```python
from build123d import *

# Parameters (mm, degrees)
F1_DEPTH = 65


# Not quite as in the source:
# - a feature names something its author has since deleted; it is built from what else it names


with BuildPart() as f1:
    # F0 (on Front) → F1 (new body)
    with BuildSketch(Plane.XZ):
        Polygon((0, 10), (0, 0), (20, 0), (20, 65), (0, 65), (0, 55), align=None)
        with BuildLine():
            ThreePointArc((13.25, 10), (10, 6.75), (6.75, 10))
            ThreePointArc((6.75, 10), (10, 13.25), (13.25, 10))
        make_face(mode=Mode.SUBTRACT)
        with BuildLine():
            ThreePointArc((13.25, 55), (10, 51.75), (6.75, 55))
            ThreePointArc((6.75, 55), (10, 58.25), (13.25, 55))
        make_face(mode=Mode.SUBTRACT)
    extrude(amount=F1_DEPTH)


solid = f1.part
```
CAD build for the part. Positions are in the model's coordinates, mm. Give positions to 0.01 mm unless a question says otherwise; leave off trailing zeros. Write each loop counter-clockwise with the first axis right and the second up, starting at its lowest first coordinate (ties: lowest second). Pieces come first, ordered by that corner, then holes. Notation, with made-up numbers: M -38.5,72 L -29.5,72 A32 ccw -29.5,108 Z; hole C 47.25,50 d5. An arc over 180 degrees is marked long. Return JSON: item names as keys, results as strings. Group by question number.
(1) Band-saw the part on B-B (y = -9). Give the cut face in (x, z), and give its area (3 significant figures).
(2) Drill centre lines: L1, parallel to Z at x = 10, y = -23.5; L2, parallel to Z at x = 12.25, y = -61.5; L3, parallel to X at y = -6, z = 13. Where is each one in solid material? Low to high. Write a range as [from, to].
(3) Mould opens along X. For faces 1 (the face through (0, -32, 33)), 2 (the face through (12.395, -32.045, 12.197)), 3 (the face through (10, -65, 33)) say: pulls with the +X half, pulls with the -X half, needs draft (parallel to the pull), parting line crosses it, or undercut.
(4) Band-saw the part on D-D (z = 57). Give the cut face in (x, y).
(5) Band-saw the part on C-C (x = 10). Give the cut face in (y, z).
(6) Band-saw the part on A-A (z = 10). Give the cut face in (x, y).
Entries:
{
 "1": {"outline": "M 0,0 L 20,0 L 20,65 L 0,65 Z; hole C 10,10 d6.5; hole C 10,55 d6.5", "area": "1,230 mm^2"},
 "2": {"L1": "z = [0, 6.75], [13.25, 51.75], [58.25, 65]", "L2": "z = [0, 7.65], [12.35, 52.65], [57.35, 65]", "L3": "x = [0, 8.75], [11.25, 20]"},
 "3": {"face 1": "pulls with the -X half", "face 2": "undercut", "face 3": "needs draft"},
 "4": {"outline": "M 0,-65 L 7.44,-65 L 7.44,0 L 0,0 Z; M 12.56,-65 L 20,-65 L 20,0 L 12.56,0 Z"},
 "5": {"outline": "M -65,0 L 0,0 L 0,6.75 L -65,6.75 Z; M -65,13.25 L 0,13.25 L 0,51.75 L -65,51.75 Z; M -65,58.25 L 0,58.25 L 0,65 L -65,65 Z"},
 "6": {"outline": "M 0,-65 L 6.75,-65 L 6.75,0 L 0,0 Z; M 13.25,-65 L 20,-65 L 20,0 L 13.25,0 Z"}
}
